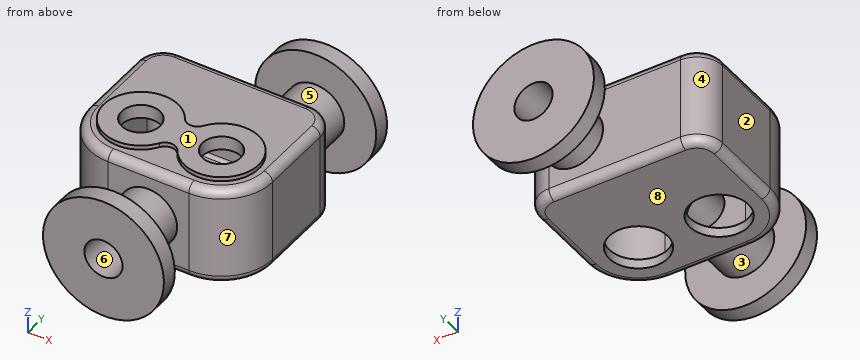
from build123d import *

# Parameters (mm, degrees)
EXTRUDE_1_DEPTH     = 46.5
FILLET_1_R          = 8
SHELL_1_T           = 9
FILLET_2_R          = 3
EXTRUDE_2_DEPTH     = 4
CUT_EXTRUDE_1_REACH = 194.273
SKETCH_3_R          = 18
CUT_EXTRUDE_2_REACH = 194.273
SKETCH_4_R          = 27.5
CUT_EXTRUDE_3_REACH = 291.997
SKETCH_7_R          = 18
CUT_EXTRUDE_4_REACH = 291.997
SKETCH_8_R          = 18


with BuildPart() as part:
    # 草圖1 → 伸長1 (new, symmetric)
    with BuildSketch(Plane.XY):
        with BuildLine():
            Line((-38, 0), (38, 0))
            ThreePointArc((38, 0), (71.941125497, 14.058874503), (86, 48))
            Line((86, 48), (86, 118))
            ThreePointArc((86, 118), (78.970562748, 134.970562748), (62, 142))
            Line((62, 142), (-62, 142))
            ThreePointArc((-62, 142), (-78.970562748, 134.970562748), (-86, 118))
            Line((-86, 118), (-86, 48))
            ThreePointArc((-86, 48), (-71.941125497, 14.058874503), (-38, 0))
        make_face()
    extrude(amount=EXTRUDE_1_DEPTH, both=True)

    # 圓角1
    fillet_1_edges = [part.edges().sort_by_distance(p)[0] for p in [
        (78.970562748, 134.970562748, 46.5),
        (0, 142, 46.5),
        (-78.970562748, 134.970562748, 46.5),
        (-86, 83, 46.5),
        (-71.941125497, 14.058874503, 46.5),
        (0, 0, 46.5),
        (71.941125497, 14.058874503, 46.5),
        (0, 0, -46.5),
        (86, 83, 46.5),
        (-71.941125497, 14.058874503, -46.5),
        (-86, 83, -46.5),
        (-78.970562748, 134.970562748, -46.5),
        (0, 142, -46.5),
        (78.970562748, 134.970562748, -46.5),
        (86, 83, -46.5),
        (71.941125497, 14.058874503, -46.5),
    ]]
    fillet(fillet_1_edges, radius=FILLET_1_R)

    # 薄殼1 (no face opened: a closed hollow body)
    add(offset(amount=-SHELL_1_T, mode=Mode.PRIVATE), mode=Mode.SUBTRACT)

    # 圓角2
    fillet_2_edges = [part.edges().sort_by_distance(p)[0] for p in [
        (65.577164466, 20.422835534, 37.5),
        (77, 83, 37.5),
        (72.606601718, 128.606601718, 37.5),
        (0, 133, -37.5),
        (-72.606601718, 128.606601718, -37.5),
        (-77, 83, -37.5),
        (-65.577164466, 20.422835534, 37.5),
        (0, 9, 37.5),
        (0, 133, 37.5),
        (-72.606601718, 128.606601718, 37.5),
        (-77, 83, 37.5),
        (72.606601718, 128.606601718, -37.5),
        (77, 83, -37.5),
        (65.577164466, 20.422835534, -37.5),
        (0, 9, -37.5),
        (-65.577164466, 20.422835534, -37.5),
    ]]
    fillet(fillet_2_edges, radius=FILLET_2_R)

    # 草圖2 → 伸長2 (add)
    with BuildSketch(Plane.XY.offset(46.5)):
        with BuildLine():
            ThreePointArc((8.444444444, 29.252489877), (73, 48), (8.444444444, 66.747510123))
            ThreePointArc((8.444444444, 66.747510123), (0, 62.103941586), (-8.444444444, 66.747510123))
            ThreePointArc((-8.444444444, 66.747510123), (-73, 48), (-8.444444444, 29.252489877))
            ThreePointArc((-8.444444444, 29.252489877), (0, 33.896058414), (8.444444444, 29.252489877))
        make_face()
    extrude(amount=EXTRUDE_2_DEPTH)

    # 草圖3 → 除料-伸長1 (cut, up to next)
    with BuildSketch(Plane.XY.offset(50.5), mode=Mode.PRIVATE) as cut_extrude_1_sk1:
        with Locations((38, 48)):
            Circle(SKETCH_3_R)
    cut_extrude_1_tool1 = extrude(cut_extrude_1_sk1.sketch, amount=-CUT_EXTRUDE_1_REACH, mode=Mode.PRIVATE) & part.part
    # 草圖3 → 除料-伸長1 (cut, up to next)
    with BuildSketch(Plane.XY.offset(50.5), mode=Mode.PRIVATE) as cut_extrude_1_sk2:
        with Locations((-38, 48)):
            Circle(SKETCH_3_R)
    cut_extrude_1_tool2 = extrude(cut_extrude_1_sk2.sketch, amount=-CUT_EXTRUDE_1_REACH, mode=Mode.PRIVATE) & part.part
    add(cut_extrude_1_tool1.solids().sort_by_distance((38, 48, 50.5))[0], mode=Mode.SUBTRACT)
    add(cut_extrude_1_tool2.solids().sort_by_distance((-38, 48, 50.5))[0], mode=Mode.SUBTRACT)

    # 草圖4 → 除料-伸長2 (cut, up to next)
    with BuildSketch(Plane(origin=(0, 0, -46.5), x_dir=(-1, 0, 0), z_dir=(0, 0, -1)), mode=Mode.PRIVATE) as cut_extrude_2_sk1:
        with Locations((-38, 48)):
            Circle(SKETCH_4_R)
    cut_extrude_2_tool1 = extrude(cut_extrude_2_sk1.sketch, amount=-CUT_EXTRUDE_2_REACH, mode=Mode.PRIVATE) & part.part
    # 草圖4 → 除料-伸長2 (cut, up to next)
    with BuildSketch(Plane(origin=(0, 0, -46.5), x_dir=(-1, 0, 0), z_dir=(0, 0, -1)), mode=Mode.PRIVATE) as cut_extrude_2_sk2:
        with Locations((38, 48)):
            Circle(SKETCH_4_R)
    cut_extrude_2_tool2 = extrude(cut_extrude_2_sk2.sketch, amount=-CUT_EXTRUDE_2_REACH, mode=Mode.PRIVATE) & part.part
    add(cut_extrude_2_tool1.solids().sort_by_distance((38, 48, -46.5))[0], mode=Mode.SUBTRACT)
    add(cut_extrude_2_tool2.solids().sort_by_distance((-38, 48, -46.5))[0], mode=Mode.SUBTRACT)

    # 草圖5 → 旋轉1 (revolve)
    with BuildSketch(Plane.XY, mode=Mode.PRIVATE) as revolve_1_sk:
        Polygon((0, -66), (57, -66), (57, -50), (27, -50), (27, 0), (0, 0), align=None)
    revolve(revolve_1_sk.sketch.rotate(Axis((0, 0, 0), (0, -1, 0)), 90), axis=Axis((0, 0, 0), (0, -1, 0)))

    # 草圖6 → 旋轉2 (revolve)
    with BuildSketch(Plane.XY, mode=Mode.PRIVATE) as revolve_2_sk:
        Polygon((11, 133), (11, 186), (-19, 186), (-19, 202), (38, 202), (38, 133), align=None)
    revolve(revolve_2_sk.sketch.rotate(Axis((38, 124.753510303, 0), (0, 1, 0)), 270), axis=Axis((38, 124.753510303, 0), (0, 1, 0)))

    # 草圖7 → 除料-伸長3 (cut, up to next)
    with BuildSketch(Plane.XZ.offset(66), mode=Mode.PRIVATE) as cut_extrude_3_sk1:
        with Locations(Location((0, 0, 0), (0, 0, 270))):
            Circle(SKETCH_7_R)
    cut_extrude_3_tool1 = extrude(cut_extrude_3_sk1.sketch, amount=-CUT_EXTRUDE_3_REACH, mode=Mode.PRIVATE) & part.part
    add(cut_extrude_3_tool1.solids().sort_by_distance((0, -66, 0))[0], mode=Mode.SUBTRACT)

    # 草圖8 → 除料-伸長4 (cut, up to next)
    with BuildSketch(Plane(origin=(0, 202, 0), x_dir=(-1, 0, 0), z_dir=(0, 1, 0)), mode=Mode.PRIVATE) as cut_extrude_4_sk1:
        with Locations(Location((-38, 0, 0), (0, 0, 90))):
            Circle(SKETCH_8_R)
    cut_extrude_4_tool1 = extrude(cut_extrude_4_sk1.sketch, amount=-CUT_EXTRUDE_4_REACH, mode=Mode.PRIVATE) & part.part
    add(cut_extrude_4_tool1.solids().sort_by_distance((38, 202, 0))[0], mode=Mode.SUBTRACT)


solid = part.part
Input: part model. Units: mm. Frame: model coordinates. Face numbers are marked on the shaded views. A direction names the side the tool comes from. Round coordinates to 2 decimals unless told otherwise and drop trailing zeros. Order: outer loops, then holes, each group sorted by start corner. A loop starts at its lowest first (then second) coordinate and runs counter-clockwise, first axis right, second up.
1. Mould query, pull axis Y, two halves, no side actions, for the marked faces 1, 2, 3 and 4. Classes: released by +Y, released by -Y, zero draft, split by the parting line, or undercut.
The answers:
face 1: undercut
face 2: zero draft
face 3: undercut
face 4: released by +Y
2. Set-up query: the marked faces 5, 6, 7 and 8. Return all of +Z, -Z, +X, -X, +Y, -Y with unobstructed straight access to the full face (end or side cutting, diameter ignored); none if empty.
The answers:
face 5: none
face 6: -Y
face 7: +Z, -Z, +X
face 8: -Z, +X, -X
3. Cut plane C-C, the plane x = -49.5. State how many separate pieces and enclosed holes the cut face has, then the cut area to 3 significant figures.
The answers:
separate pieces: 3
enclosed holes: 0
area: 4,220 mm2
4. Pin query (flat end, axial travel): P1, Ø10, axis at x = 63, z = 32.5, coming from the -Y side; P2, Ø10, axis at y = 163.5, z = 15, coming from the +X side; P3, Ø3, axis at x = 21, y = 108, coming from the -Z side; P4, Ø23, axis at x = -27.5, z = 8, coming from the +Y side. Return the tip coordinate at first contact, or that it passes through.
The answers:
P1: stops at y = 4.37
P2: stops at x = 63.08
P3: stops at z = -46.5
P4: stops at y = 202
5. Cut plane A-A, the plane z = 30.5. Output: boundary loops of the cut face in (x, y).
The answers:
outline: (-86, 48) arc R48 ccw to (-38, 0) - (38, 0) arc R48 ccw to (86, 48) - (86, 118) arc R24 ccw to (62, 142) - (-62, 142) arc R24 ccw to (-86, 118) - close; (-48.15, -66) - (48.15, -66) - (48.15, -50) - (-48.15, -50) - close; (-10.15, 186) - (86.15, 186) - (86.15, 202) - (-10.15, 202) - close; hole (-77, 48) arc R39 ccw to (-38, 9) - (38, 9) arc R39 ccw to (77, 48) - (77, 118) arc R15 ccw to (62, 133) - (-62, 133) arc R15 ccw to (-77, 118) - close
6. Cut plane B-B, the plane y = -25. Output: boundary loops of the cut face in (x, z).
The answers:
outline: circle Ø54 at (0, 0); hole circle Ø36 at (0, 0)
7. Material intervals for line 1 (Y direction, x = -6, z = -29.5); line 2 (Z direction, x = 7, y = 95); line 3 (Z direction, x = 19.5, y = 74.5), sorted ascending.
The answers:
line 1: y = -66 to -50, 0 to 9, 133 to 142, 186 to 202
line 2: z = -46.5 to -37.5, 37.5 to 46.5
line 3: z = -46.5 to -37.5, 37.5 to 50.5
